from build123d import *

# Parameters (mm, degrees)
F0_W     = 127
F0_H     = 12.7
F1_DEPTH = 63.5
F0_H_2   = 76.9474954844
F0_H_3   = 11.9525045156
F2_DEPTH = 6.35
F3_W     = 127
F3_H     = 3.8452798724
F4_DEPTH = 50.8
F5_R     = 5.08


with BuildPart() as f1:
    # F0 (on Front) → F1 (new body)
    with BuildSketch(Plane.XZ):
        with Locations((7.5608139634, -7.8621631652)):
            Rectangle(F0_W, F0_H)
    extrude(amount=F1_DEPTH)

    # F0 (on Front) → F2 (join)
    with BuildSketch(Plane.XZ):
        with Locations((7.5608139634, 36.961584577)):
            Rectangle(F0_W, F0_H_2)
        with Locations((7.5608139634, -20.188415423)):
            Rectangle(F0_W, F0_H_3)
        with Locations((7.5608139634, -7.8621631652)):
            Rectangle(F0_W, F0_H)
    extrude(amount=F2_DEPTH)

    # F3 (on face) → F4 (join)
    with BuildSketch(Plane.XY.offset(-1.5121631652)):
        with Locations((7.5608139634, -61.5773600638)):
            Rectangle(F3_W, F3_H)
    extrude(amount=F4_DEPTH)

    # F5
    f5_edges = [f1.edges().sort_by_distance(p)[0] for p in [
        (7.560814, -63.5, -14.212163),
        (71.060814, -34.925, -14.212163),
        (7.560814, -6.35, -26.164668),
        (-55.939186, -6.35, -20.188415),
        (-55.939186, -34.925, -14.212163),
        (71.060814, -6.35, -20.188415),
        (7.560814, -6.35, -14.212163),
        (-55.939186, -6.35, 36.961585),
        (7.560814, -6.35, -1.512163),
        (7.560814, -6.35, 75.435332),
        (71.060814, -33.00236, -1.512163),
        (71.060814, -6.35, 36.961585),
        (-55.939186, -33.00236, -1.512163),
    ]]
    fillet(f5_edges, radius=F5_R)


solid = f1.part
Verification items for the finished model (mm, model axes). A direction names the side the tool comes from. Coordinates: 2 decimals unless noted, no trailing zeros. Order: outer loops, then holes, each group sorted by start corner. A loop starts at its lowest first (then second) coordinate and runs counter-clockwise, first axis right, second up. Notation, with made-up numbers: M 15.25,0.5 L 55.25,0.5 A23 cw 55.25,29.5 Z; hole C 69,-9 d7. An arc over 180 degrees is marked long. Return JSON: item names as keys, results as strings.
1) Cross-section at C-C, the plane y = -43. Record the boundary of the cut face in (x, z).
Answer list:
{"outline": "M -55.94,-9.13 A5.08 ccw -50.86,-14.21 L 65.98,-14.21 A5.08 ccw 71.06,-9.13 L 71.06,-6.59 A5.08 ccw 65.98,-1.51 L -50.86,-1.51 A5.08 ccw -55.94,-6.59 Z"}
2) Access from +Z, -Z, +X, -X, +Y, -Y to the whole of each face (thin tool, end or side, straight path). Record for faces 4 (the flat face through (7, -62, 49.288)), 5 (the cylindrical face through (-54.491, -37.829, -12.685)), 6 (the cylindrical face through (8.379, -7.799, 0.015)), 7 (the cylindrical face through (-54.491, -4.822, 38.999)), 8 (the cylindrical face through (69.612, -37.829, -12.685)).
Answer list:
{"face 4": "+Z, +X, -X, -Y", "face 5": "-Z, -X, -Y", "face 6": "+Z, +X, -X", "face 7": "+Z, -X", "face 8": "-Z, +X, -Y"}
3) Release check for a two-part mould opening along Y. For faces 1 (the cylindrical face through (8.45, -4.9, -24.64)), 2 (the flat face through (7, -35, -14.212)), 3 (the flat face through (7, -6.35, 37)) record: +Y half, -Y half, draft (parallel to the pull), parting line (faces both ways), or undercut.
Answer list:
{"face 1": "-Y half", "face 2": "draft", "face 3": "undercut"}
4) Cross-section at D-D, the plane z = 61. Record the boundary of the cut face in (x, y), and give its area (3 significant figures).
Answer list:
{"outline": "M -55.94,-1.27 A5.08 ccw -50.86,-6.35 L 65.98,-6.35 A5.08 ccw 71.06,-1.27 L 71.06,0 L -55.94,0 Z", "area": "795 mm2"}
5) Cross-section at B-B, the plane x = 26. Record the boundary of the cut face in (y, z), and give its area (3 significant figures).
Answer list:
{"outline": "M -63.5,-9.13 A5.08 ccw -58.42,-14.21 L -11.43,-14.21 A5.08 cw -6.35,-19.29 L -6.35,-21.08 A5.08 ccw -1.27,-26.16 L 0,-26.16 L 0,75.44 L -1.27,75.44 A5.08 ccw -6.35,70.36 L -6.35,3.57 A5.08 cw -11.43,-1.51 L -59.65,-1.51 L -59.65,49.29 L -63.5,49.29 Z", "area": "1,560 mm2"}
6) Thickness scan on L1, parallel to Y at x = 46, z = 29; L2, parallel to Z at x = -30, y = -59; L3, parallel to Y at x = 40.5, z = -20.5. Record the ranges inside material, lowest first. Write a range as [from, to].
Answer list:
{"L1": "[-63.5, -59.65], [-6.35, 0]", "L2": "[-14.18, -1.51]", "L3": "[-6.35, 0]"}
7) Gauge pin test, flat ends, axial feed: pin 1 (5 mm diameter, centred on y = -20, z = -15.5, fed in from +X); pin 2 (4 mm diameter, centred on x = 0.5, z = 63, fed in from -Y); pin 3 (10 mm diameter, centred on x = -0.5, y = -24.5, fed in from -Z). Record the tip position at first contact, or that the pin passes through.
Answer list:
{"pin 1": "x = 69.27", "pin 2": "y = -6.35", "pin 3": "z = -14.21"}
8) Cross-section at A-A, the plane z = 27. Record the boundary of the cut face in (x, y).
Answer list:
{"outline": "M -55.94,-63.5 L 71.06,-63.5 L 71.06,-59.65 L -55.94,-59.65 Z; M -55.94,-1.27 A5.08 ccw -50.86,-6.35 L 65.98,-6.35 A5.08 ccw 71.06,-1.27 L 71.06,0 L -55.94,0 Z"}
